Design review of the part built by this model. Coordinates are the model's own, in mm. A direction names the side the tool comes from. Round coordinates to 2 decimals unless told otherwise and drop trailing zeros. Loops run counter-clockwise (first coordinate to the right, second up) from the corner with the lowest first, then second, coordinate; pieces in that order, holes last. Notation, with made-up numbers: (51.25, 56.5) -> (60.25, 56.5) arc R30 cw to (60.25, 81.5) -> close; hole circle Ø6 at (79, -20). An arc over 180 degrees is marked (long way). Answer as CSV lines item,"result". Start each with the question number.
Autodesk Inventor part; units mm, degrees
ref_plane "YZ Plane" through (0, 0, 0) normal (1, 0, 0) x (0, 1, 0)
ref_plane "XZ Plane" through (0, 0, 0) normal (0, 1, 0) x (-1, 0, 0)
ref_plane "XY Plane" through (0, 0, 0) normal (0, 0, 1) x (1, 0, 0)
sketch "Sketch1" plane through (0, 0, 0) normal (0, 1, 0) x (-1, 0, 0)
  line L0 (0, 0) -> (35, 0)
  line L1 (35, 0) -> (35, -16)
  line L2 (35, -16) -> (32, -16)
  line L3 (32, -16) -> (32, -14)
  line L4 (32, -14) -> (0, -14)
  line L5 (0, -14) -> (0, 0)
  line L6 (35, 0) -> (45, 0)
  line L7 (45, 0) -> (45, -11)
  line L8 (45, -11) -> (35, -11)
  line L9 (5, 0) -> (5, -11)
  line L10 (5, -11) -> (45, -11)
  line L11 (27, -14) -> (27, -12.8)
  line L12 (27, -12.8) -> (29, -12.8)
  line L13 (29, -12.8) -> (29, -14)
  line L14 (45, -11) -> (55, -11)
  line L15 (55, -11) -> (55, -13.5)
  line L16 (55, -13.5) -> (35, -13.5)
  point P0 (35, -11)
  point P1 (32, -15)
  point P2 (27, -11)
  point P3 (29, -11)
  dimension "d0" = 28
  dimension "d1" = 32
  dimension "d2" = 3
  dimension "d3" = 35
  dimension "d5" = 10
  dimension "d6" = 5
  dimension "d7" = 3
  dimension "d18" = 2
  dimension "d20" = 22
  dimension "d21" = 3
  dimension "d24" = 1.2
  dimension "d25" = 50
  dimension "d26" = 2.5
revolve "Revolution1" add sketch "Sketch1" angle 360 about axis through (0, 0, 0) along (-1, 0, 0) contours L0 L9 L10 L1 L2 L3 L4 L13 L12 L11 L5 | L8 L14 L15 L16 L1
sketch "Sketch2" plane through (0, 0, 0) normal (1, 0, 0) x (0, 0, -1)
  point P0 (0, 0)
  point P1 (0, 0)
  point P2 (6, 0)
  point P3 (-6, 0)
  point P4 (0, 6)
  dimension "d22" = 6
  dimension "d23" = 6
  dimension "d27" = 6
hole "Hole1" at (0, 0, -6) at (0, 0, 6) at (0, 6, 0) direction (-1, 0, 0) diameter 3.4 end through all
sketch "Sketch3" plane through (-5, 0, 0) normal (-1, 0, 0) x (0, 0, 1)
  circle A0 centre (0, 6) radius 1.7
  circle A1 centre (-6, 0) radius 1.7
  circle A2 centre (6, 0) radius 1.7
  circle A3 centre (6, 0) radius 3.75
  circle A4 centre (0, 6) radius 3.75
  circle A5 centre (-6, 0) radius 3.75
  circle A6 centre (6, 0) radius 1.7
  circle A7 centre (-6, 0) radius 1.7
  circle A8 centre (0, 6) radius 1.7
  circle A9 centre (0, 0) radius 11
  dimension "d28" = 7.5
  dimension "d29" = 7.5
  dimension "d30" = 7.5
extrude "Extrusion1" add sketch "Sketch3" along normal blind 10 contours A9
properties part number "028" material "PC/ABS Plastic"
Q1. For pin 1 Ø8 at (y, z) = (0.5, 7.5) entering from -X; pin 2 Ø1.5 at (y, z) = (5.5, -0.5) entering from -X; pin 3 Ø11 at (y, z) = (0.5, 4.5) entering from -X; pin 4 Ø6 at (y, z) = (0, -6) entering from -X, all flat-tipped, find the tip position at first contact; note any pin that passes through.
Q2. Machinability: for faces 4 (the flat face through (-55, 10, 5)), 5 (the cylindrical face through (-35.28, 10.74, 2.38)), 6 (the flat face through (-32, 14.15, 0.07)), which of the approach directions +Z, -Z, +X, -X, +Y, -Y give a long, thin tool a straight path to every point of the face, cutting with its end or side? Answer none if there is none.
Q3. Add section C-C, the plane x = -42.5. Give the boundary of the cut face in (y, z), and give its area (3 significant figures).
Q4. To check wall thickness, follow probe 1 along Z at (x, y) = (-1.9, 0); probe 2 along Z at (x, y) = (-10.5, -2.5); probe 3 along X at (y, z) = (-13, -1). State the ranges of each line that lie inside material, in increasing order. Write a range as from..to.
Q5. Add section D-D, the plane y = -5. Give the boundary of the cut face in (x, z), and give its area (3 significant figures).
Q6. Mouldability with a two-part tool opening along Z and no side actions: class faces 1 (the flat face through (-27, 4.1, -12.4)), 2 (the cylindrical face through (-13.311, -5.362, -12.932)), 3 (the cylindrical face through (-9.93, -0.165, 2.254)) as pulls with the +Z half, pulls with the -Z half, needs draft (parallel to the pull), parting line crosses it, or undercut.
Worked answers:
1,pin 1,"stops at x = -55"
1,pin 2,"passes through"
1,pin 3,"stops at x = -15"
1,pin 4,"stops at x = -5"
2,face 4,"+Z, -Z, -X, +Y, -Y"
2,face 5,"-X"
2,face 6,"+X"
3,outline,"circle Ø27 at (0, 0); hole circle Ø22 at (0, 0)"
3,area,"192 mm^2"
4,probe 1,"z = -14..-7.7, -4.3..4.3, 7.7..14"
4,probe 2,"z = -13.77..-8.8, -3.2..3.2, 8.8..13.77"
4,probe 3,"x = -55..-29, -27..0"
5,outline,"(-55, -12.54) -> (-35, -12.54) -> (-35, -15.2) -> (-32, -15.2) -> (-32, -13.08) -> (-29, -13.08) -> (-29, -11.78) -> (-27, -11.78) -> (-27, -13.08) -> (0, -13.08) -> (0, 13.08) -> (-27, 13.08) -> (-27, 11.78) -> (-29, 11.78) -> (-29, 13.08) -> (-32, 13.08) -> (-32, 15.2) -> (-35, 15.2) -> (-35, 12.54) -> (-55, 12.54) -> (-55, 9.8) -> (-15, 9.8) -> (-15, -9.8) -> (-55, -9.8) -> close"
5,area,"641 mm^2"
6,face 1,"needs draft"
6,face 2,"parting line crosses it"
6,face 3,"undercut"
